Check sheet for the modelled part. Datum: model origin and axes. Units: mm. Face numbers are marked on the shaded views. A direction names the side the tool comes from. Coordinates: 2 decimals unless noted, no trailing zeros. Write each loop counter-clockwise with the first axis right and the second up, starting at its lowest first coordinate (ties: lowest second). Pieces come first, ordered by that corner, then holes. Notation, with made-up numbers: (44.25, 70.5) -> (67.25, 70.5) arc R26 ccw to (67.25, 93.5) -> close; hole circle Ø2 at (43, -29.5). An arc over 180 degrees is marked (long way). Put each result on its own line as item: value.
```python
from build123d import *

# Parameters (mm, degrees)
SKETCH1_W                                      = 52
SKETCH1_H                                      = 45
BOSS_EXTRUDE1_DEPTH                            = 15
SKETCH2_R                                      = 11.5
CUT_EXTRUDE1_DEPTH                             = 2
CBORE_FOR_4_SOCKET_HEAD_CAP_SCREW1_D           = 3.2639
CBORE_FOR_4_SOCKET_HEAD_CAP_SCREW1_CBORE_D     = 5.55752
CBORE_FOR_4_SOCKET_HEAD_CAP_SCREW1_CBORE_DEPTH = 2.8448
CUT_EXTRUDE3_DEPTH                             = 71.384657419
CUT_EXTRUDE4_DEPTH                             = 10
CUT_EXTRUDE5_DEPTH                             = 6
M5_TAPPED_HOLE3_D                              = 4.2


with BuildPart() as part:
    # Sketch1 → Boss-Extrude1 (new body)
    with BuildSketch(Plane(origin=(0, 0, 0), x_dir=(1, 0, 0), z_dir=(0, 1, 0))):
        with Locations((26, 22.5)):
            Rectangle(SKETCH1_W, SKETCH1_H)
    extrude(amount=BOSS_EXTRUDE1_DEPTH)

    # Sketch2 → Cut-Extrude1 (cut)
    with BuildSketch(Plane.XZ):
        with Locations(Location((33.048851489, -22.5, 0), (0, 0, 270))):
            Circle(SKETCH2_R)
    extrude(amount=-CUT_EXTRUDE1_DEPTH, mode=Mode.SUBTRACT)

    # CBORE for _4 Socket Head Cap Screw1 (through all)
    with Locations(Plane(origin=(0, 15, 0), x_dir=(-1, 0, 0), z_dir=(0, 1, 0))):
        with Locations((-48.548851489, -38), (-48.548851489, -7), (-17.548851489, -7), (-17.548851489, -38)):
            CounterBoreHole(CBORE_FOR_4_SOCKET_HEAD_CAP_SCREW1_D / 2, CBORE_FOR_4_SOCKET_HEAD_CAP_SCREW1_CBORE_D / 2, CBORE_FOR_4_SOCKET_HEAD_CAP_SCREW1_CBORE_DEPTH)

    # Sketch8 → Cut-Extrude3 (cut, through all)
    with BuildSketch(Plane(origin=(0, 15, 0), x_dir=(1, 0, 0), z_dir=(0, 1, 0))):
        with BuildLine():
            Line((27.048851489, 22.5), (27.048851489, 27.869202711))
            ThreePointArc((27.048851489, 27.869202711), (24.562140957, 34.365125617), (27.7583836, 40.542890313))
            Line((27.7583836, 40.542890313), (30.889155511, 43.032522261))
            ThreePointArc((30.889155511, 43.032522261), (42.879465836, 41.610512499), (41.350499943, 29.633371074))
            Line((41.350499943, 29.633371074), (39.048851489, 27.869202711))
            Line((39.048851489, 27.869202711), (39.048851489, 22.5))
            ThreePointArc((39.048851489, 22.5), (33.048851489, 16.5), (27.048851489, 22.5))
        make_face()
    extrude(amount=-CUT_EXTRUDE3_DEPTH, mode=Mode.SUBTRACT)

    # Sketch11 → Cut-Extrude4 (cut)
    with BuildSketch(Plane(origin=(0, 15, 0), x_dir=(1, 0, 0), z_dir=(0, 1, 0))):
        with BuildLine():
            Line((23.601490667, 12.384290412), (23.601490667, 3.652513208))
            ThreePointArc((23.601490667, 3.652513208), (24.333723714, 1.884746256), (26.101490667, 1.152513208))
            Line((26.101490667, 1.152513208), (41.505460803, 1.152513208))
            ThreePointArc((41.505460803, 1.152513208), (43.273227756, 1.884746256), (44.005460803, 3.652513208))
            Line((44.005460803, 3.652513208), (44.005460803, 13.09315188))
            ThreePointArc((44.005460803, 13.09315188), (43.852771156, 13.953462349), (43.41335352, 14.708684417))
            Line((43.41335352, 14.708684417), (39.048851489, 19.863022972))
            Line((39.048851489, 19.863022972), (39.048851489, 34.725308874))
            Line((39.048851489, 34.725308874), (27.048851489, 34.725308874))
            Line((27.048851489, 34.725308874), (27.048851489, 22.5))
            ThreePointArc((27.048851489, 22.5), (27.839413547, 19.523129776), (30.002770266, 17.330726436))
            Line((30.002770266, 17.330726436), (30.002770266, 14.884290412))
            Line((30.002770266, 14.884290412), (26.101490667, 14.884290412))
            ThreePointArc((26.101490667, 14.884290412), (24.333723714, 14.152057365), (23.601490667, 12.384290412))
        make_face()
    extrude(amount=-CUT_EXTRUDE4_DEPTH, mode=Mode.SUBTRACT)

    # Sketch12 → Cut-Extrude5 (cut)
    with BuildSketch(Plane(origin=(0, 15, 0), x_dir=(1, 0, 0), z_dir=(0, 1, 0))):
        Polygon((43.546506973, 11.676957706), (53.351680383, 11.676957706), (53.351680383, 20.978390716), (41.522528086, 35.389540724), (36.326040528, 27.362061402), (38.483158835, 17.285853694), align=None)
    extrude(amount=-CUT_EXTRUDE5_DEPTH, mode=Mode.SUBTRACT)

    # M5 Tapped Hole3 (through all)
    with Locations(Plane(origin=(0, 15, 0), x_dir=(-1, 0, 0), z_dir=(0, 1, 0))):
        with Locations((-47, -19.55942237)):
            Hole(M5_TAPPED_HOLE3_D / 2)


solid = part.part
```
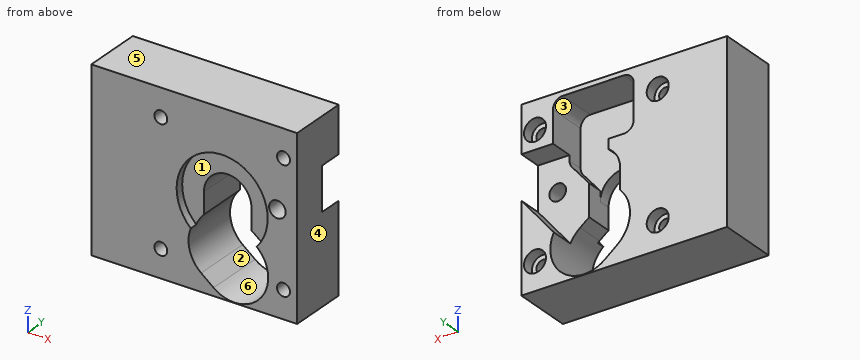
Q1. Cross-section at B-B (y = 13.5). Record the cut outline in (x, z), plus the area to 3 significant figures.
Recorded:
outline: (0, -45) -> (52, -45) -> (52, -22.63) -> (43.8, -32.61) arc R8.5 cw to (30.89, -43.03) -> (27.76, -40.54) arc R8.5 cw to (27.05, -27.87) -> (27.05, -22.5) arc R6 cw to (30, -17.33) -> (30, -14.88) -> (26.1, -14.88) arc R2.5 cw to (23.6, -12.38) -> (23.6, -3.65) arc R2.5 cw to (26.1, -1.15) -> (41.51, -1.15) arc R2.5 cw to (44.01, -3.65) -> (44.01, -11.68) -> (52, -11.68) -> (52, 0) -> (0, 0) -> close; hole circle Ø5.56 at (17.55, -38); hole circle Ø5.56 at (17.55, -7); hole circle Ø5.56 at (48.55, -38); hole circle Ø5.56 at (48.55, -7)
area: 1,350 mm2
Q2. Depth check by flat-ended pin: P1, Ø10, axis at x = 37.5, z = -9.5, coming from the +Y side; P2, Ø5, axis at x = 48.55, z = -7, coming from the +Y side. Enter the tip coordinate at first touch or a pass-through.
Recorded:
P1: stops at y = 5
P2: stops at y = 12.16
Q3. Cross-section at A-A (z = -7). Record the cut outline in (x, y).
Recorded:
outline: (0, 0) -> (15.92, 0) -> (15.92, 12.16) -> (14.77, 12.16) -> (14.77, 15) -> (0, 15) -> close; (19.18, 0) -> (46.92, 0) -> (46.92, 12.16) -> (45.77, 12.16) -> (45.77, 15) -> (44.01, 15) -> (44.01, 5) -> (23.6, 5) -> (23.6, 15) -> (20.33, 15) -> (20.33, 12.16) -> (19.18, 12.16) -> close; (50.18, 0) -> (52, 0) -> (52, 15) -> (51.33, 15) -> (51.33, 12.16) -> (50.18, 12.16) -> close
Q4. Cross-section at C-C (z = -28.5). Record the cut outline in (x, y).
Recorded:
outline: (0, 0) -> (23.24, 0) -> (23.24, 2) -> (26.48, 2) -> (26.48, 15) -> (0, 15) -> close; (39.87, 2) -> (42.86, 2) -> (42.86, 0) -> (52, 0) -> (52, 15) -> (47.18, 15) -> (47.18, 9) -> (39.87, 9) -> close
Q5. Mould release check, pull along X, two halves, no side actions. Record for the marked faces 4, 5 and 6: released by +X, released by -X, zero draft, split by the parting line, or undercut.
Recorded:
face 4: released by +X
face 5: zero draft
face 6: undercut
Q6. Material ranges on line 1 along X through (y, z) = (8.5, -26); line 2 along X through (y, z) = (5.75, -10); line 3 along X through (y, z) = (3.25, -37), recorded low to high.
Recorded:
line 1: x = 0 to 27.05, 39.05 to 52
line 2: x = 0 to 23.6, 44.01 to 52
line 3: x = 0 to 16.26, 18.84 to 25.14, 44.66 to 47.26, 49.84 to 52
Q7. Cross-section at D-D (x = 48.5). Record the cut outline in (y, z), plus the area to 3 significant figures.
Recorded:
outline: (0, -45) -> (15, -45) -> (15, -40.78) -> (12.16, -40.78) -> (12.16, -39.63) -> (0, -39.63) -> close; (0, -36.37) -> (12.16, -36.37) -> (12.16, -35.22) -> (15, -35.22) -> (15, -26.89) -> (9, -26.89) -> (9, -21.03) -> (0, -21.03) -> close; (0, -18.09) -> (9, -18.09) -> (9, -11.68) -> (15, -11.68) -> (15, -9.78) -> (12.16, -9.78) -> (12.16, -8.63) -> (0, -8.63) -> close; (0, -5.37) -> (12.16, -5.37) -> (12.16, -4.22) -> (15, -4.22) -> (15, 0) -> (0, 0) -> close
area: 446 mm2
Q8. Tool access check on the marked faces 1, 2 and 3. Record the directions out of +Z, -Z, +X, -X, +Y, -Y that give a thin tool (end or side, any length) a straight path to the whole face; none if there is none.
Recorded:
face 1: -Y
face 2: +Y, -Y
face 3: +Y
